Drawing for the job (mm, zero at the part's lowest x, y, z). Give positions to 0.01 mm unless a question says otherwise; leave off trailing zeros. Order: outer loops, then holes, each group sorted by start corner. A loop starts at its lowest first (then second) coordinate and runs counter-clockwise, first axis right, second up. Notation, with made-up numbers: (33.5, 2) - (40.5, 2) arc R29 ccw to (40.5, 36) - close; hole circle Ø11 at (79.5, -3). An arc over 180 degrees is marked (long way). One line per item, written item: value.
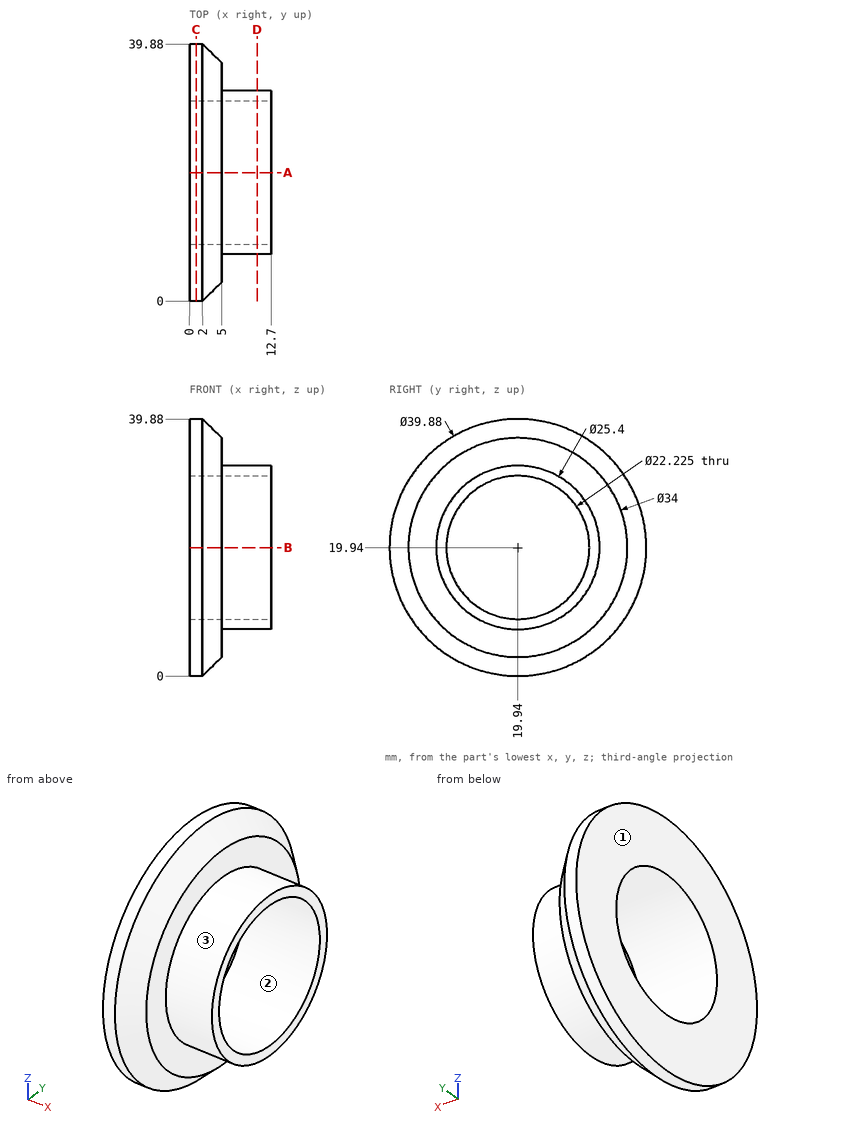
(1) Slice it at A-A, the plane y = 19.94. Give the cut face in (x, z), and give its area (3 significant figures).
Completed:
outline: (0, 0) - (2, 0) - (5, 2.94) - (5, 7.24) - (12.7, 7.24) - (12.7, 8.83) - (0, 8.83) - close; (0, 31.05) - (12.7, 31.05) - (12.7, 32.64) - (5, 32.64) - (5, 36.94) - (2, 39.88) - (0, 39.88) - close
area: 104 mm²
(2) Pull direction Z, two halves, no side cores. Call the marked faces 1, 2 and 3: +Z half, -Z half, draft (parallel to the pull), parting line (faces both ways), or undercut.
Completed:
face 1: draft
face 2: undercut
face 3: parting line
(3) Drill centre lines: line 1 (Z direction, x = 5.25, y = 19.94); line 2 (Y direction, x = 7.5, z = 10). Where is each one in solid material? Low to high.
Completed:
line 1: 7.24 to 8.83, 31.05 to 32.64
line 2: 12.04 to 14.97, 24.91 to 27.84
(4) Pin check, flat tips, straight feed: P1, Ø5, axis at x = 4, y = 12, coming from the +Z side; P2, Ø1.5, axis at x = 2.5, y = 33.5, coming from the +Z side; P3, Ø6, axis at x = 4.5, z = 15, coming from the -Y side; P4, Ø20, axis at y = 19.94, z = 19.94, coming from the -X side. Stop position of each tip, or through.
Completed:
P1: z = 38.81
P2: z = 35.06
P3: y = 0.27
P4: through
(5) Slice it at C-C, the plane x = 1. Give the cut face in (y, z) (1 decimal).
Completed:
outline: circle Ø39.9 at (19.9, 19.9); hole circle Ø22.2 at (19.9, 19.9)
(6) Slice it at D-D, the plane x = 10.5. Give the cut face in (y, z) (1 decimal), and give its area (3 significant figures).
Completed:
outline: circle Ø25.4 at (19.9, 19.9); hole circle Ø22.2 at (19.9, 19.9)
area: 119 mm²
